Verification items for the finished model (mm, model axes). A direction names the side the tool comes from. Round coordinates to 2 decimals unless told otherwise and drop trailing zeros. Loops run counter-clockwise (first coordinate to the right, second up) from the corner with the lowest first, then second, coordinate; pieces in that order, holes last. Notation, with made-up numbers: M 30,65 L 79,65 A30 cw 79,91 Z; hole C -27,75.5 d1. An arc over 180 degrees is marked long. Write item = value, one per line. Start each with the question number.
from build123d import *

# Parameters (mm, degrees)
F0_W     = 31.1
F0_H     = 15.8
F1_DEPTH = 20.2
F0_H_2   = 21.8
F2_DEPTH = 4.7
F3_R     = 5.25
F4_DEPTH = 37.601
F5_R     = 3.35
F6_DEPTH = 4.701
F7_R     = 4.5
F8_DEPTH = 9


with BuildPart() as f1:
    # F0 (on Top) → F1 (new body)
    with BuildSketch(Plane.XY):
        with Locations((15.55, 7.9)):
            Rectangle(F0_W, F0_H)
    extrude(amount=F1_DEPTH)

    # F0 (on Top) → F2 (join)
    with BuildSketch(Plane.XY):
        with Locations((15.55, 7.9)):
            Rectangle(F0_W, F0_H)
        with Locations((15.55, 26.7)):
            Rectangle(F0_W, F0_H_2)
    extrude(amount=F2_DEPTH)

    # F3 (on face) → F4 (cut, through all)
    with BuildSketch(Plane.XZ):
        with Locations((7.85, 10.25)):
            Circle(F3_R)
        with Locations((23.25, 10.25)):
            Circle(F3_R)
    extrude(amount=-F4_DEPTH, mode=Mode.SUBTRACT)

    # F5 (on face) → F6 (cut, through all)
    with BuildSketch(Plane.XY.offset(4.7)):
        with Locations((15.55, 26.35)):
            Circle(F5_R)
    extrude(amount=-F6_DEPTH, mode=Mode.SUBTRACT)

    # F7 (on face) → F8 (cut)
    with BuildSketch(Plane.XY.offset(20.2)):
        with Locations((7.75, 7.75)):
            Circle(F7_R)
        with Locations((23.35, 7.75)):
            Circle(F7_R)
    extrude(amount=-F8_DEPTH, mode=Mode.SUBTRACT)


solid = f1.part
1. Section check C-C, the plane y = 2. Enter the section's corners in (x, z).
2. Mould release check, pull along X, two halves, no side actions. Record for faces 3 (the cylindrical face through (4.18, 5.01, 17.37)), 4 (the cylindrical face through (25.769, 11.544, 17.367)), 5 (the flat face through (0, 10, 8)), 6 (the flat face through (15, 19, 0)): pulls with the +X half, pulls with the -X half, needs draft (parallel to the pull), parting line crosses it, or undercut.
3. Tool access check on faces 1 (the cylindrical face through (12.203, 26.497, 2.383)), 2 (the flat face through (15, 15.8, 14)). Record the directions out of +Z, -Z, +X, -X, +Y, -Y that give a thin tool (end or side, any length) a straight path to the whole face; none if there is none.
4. Section check D-D, the plane x = 7.75. Enter the section's corners in (y, z).
5. Section check B-B, the plane y = 26.35. Enter the section's corners in (x, z).
6. Gauge pin test, flat ends, axial feed: P1, Ø5.5, axis at x = 23.35, y = 7.75, coming from the +Z side; P2, Ø5, axis at x = 13.5, z = 15, coming from the +Y side; P3, Ø4, axis at x = 19.5, y = 31.5, coming from the +Z side. Record the tip position at first contact, or that the pin passes through.
7. Section check A-A, the plane z = 10.25. Enter the section's corners in (x, y).
8. Thickness scan on line 1 (X direction, y = 7.75, z = 14.5); line 2 (X direction, y = 14.5, z = 12.75); line 3 (Y direction, x = 7.75, z = 18.25). Record the ranges inside material, lowest first.
Computed values:
q1.outline = M 0,0 L 31.1,0 L 31.1,20.2 L 0,20.2 Z; hole C 7.85,10.25 d10.5; hole C 23.25,10.25 d10.5
q2.face_3 = undercut
q2.face_4 = undercut
q2.face_5 = pulls with the -X half
q2.face_6 = needs draft
q3.face_1 = +Z, -Z
q3.face_2 = +Z, +X, -X, +Y
q4.outline = M 0,0 L 37.6,0 L 37.6,4.7 L 15.8,4.7 L 15.8,5 L 0,5 Z; M 0,15.5 L 3.25,15.5 L 3.25,20.2 L 0,20.2 Z; M 12.25,15.5 L 15.8,15.5 L 15.8,20.2 L 12.25,20.2 Z
q5.outline = M 0,0 L 12.2,0 L 12.2,4.7 L 0,4.7 Z; M 18.9,0 L 31.1,0 L 31.1,4.7 L 18.9,4.7 Z
q6.P1 = 5.84
q6.P2 = 15.8
q6.P3 = 4.7
q7.outline = M 0,0 L 2.6,0 L 2.6,15.8 L 0,15.8 Z; M 13.1,0 L 18,0 L 18,15.8 L 13.1,15.8 Z; M 28.5,0 L 31.1,0 L 31.1,15.8 L 28.5,15.8 Z
q8.line_1 = 0 to 3.25, 12.25 to 18.85, 27.85 to 31.1
q8.line_2 = 0 to 3.23, 12.47 to 18.63, 27.87 to 31.1
q8.line_3 = 0 to 3.25, 12.25 to 15.8
